Work out the finished part from the listing and answer in its coordinate system (mm). Round coordinates to 2 decimals unless told otherwise and drop trailing zeros. Order: outer loops, then holes, each group sorted by start corner. A loop starts at its lowest first (then second) coordinate and runs counter-clockwise, first axis right, second up.
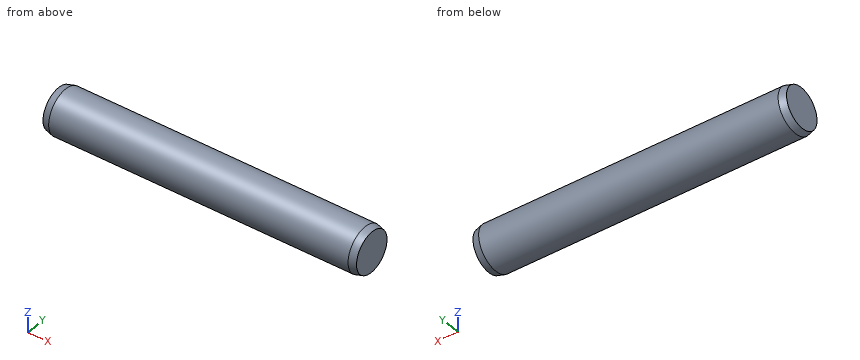
from build123d import *

# Parameters (mm, degrees)
SKETCH2_R           = 2
EXTRUDE1_DEPTH      = 13.37
EXTRUDE1_DEPTH_BACK = 13.37
SKETCH3_R           = 2
EXTRUDE2_DEPTH      = 0.63
EXTRUDE2_TAPER      = 15
SKETCH4_R           = 2
EXTRUDE3_DEPTH      = 0.63
EXTRUDE3_TAPER      = 15


with BuildPart() as part:
    # Sketch2 → Extrude1 (new body, two sides)
    with BuildSketch(Plane(origin=(0, 0, 0), x_dir=(0, 0, -1), z_dir=(1, 0, 0))) as extrude1_sk:
        Circle(SKETCH2_R)
    extrude(amount=EXTRUDE1_DEPTH)
    extrude(extrude1_sk.sketch, amount=-EXTRUDE1_DEPTH_BACK)

    # Sketch3 → Extrude2 (add)
    with BuildSketch(Plane(origin=(13.37, 0, 0), x_dir=(0, 0, -1), z_dir=(1, 0, 0))):
        Circle(SKETCH3_R)
    extrude(amount=EXTRUDE2_DEPTH, taper=EXTRUDE2_TAPER)

    # Sketch4 → Extrude3 (add)
    with BuildSketch(Plane.ZY.offset(13.37)):
        Circle(SKETCH4_R)
    extrude(amount=EXTRUDE3_DEPTH, taper=EXTRUDE3_TAPER)


solid = part.part
Item 1: Find section A-A (x = -3). Write down the section's boundary in (y, z).
Item 2: Find the intervals of material crossed by line 1 along Z through (x, y) = (-13, -1.25); line 2 along Y through (x, z) = (-1.25, 1.8); line 3 along Y through (x, z) = (3.25, 0.35), in increasing order.
Item 3: Given pin 1 (1.5 mm diameter, centred on x = 3, z = 1.5, fed in from +Y), flat-ended and moving along its own axis, determine where the tip first touches the part or whether it passes through.
Model answer:
1. outline: circle Ø4 at (0, 0)
2. line 1: z = -1.56 to 1.56
2. line 2: y = -0.87 to 0.87
2. line 3: y = -1.97 to 1.97
3. pin 1: stops at y = 1.85
